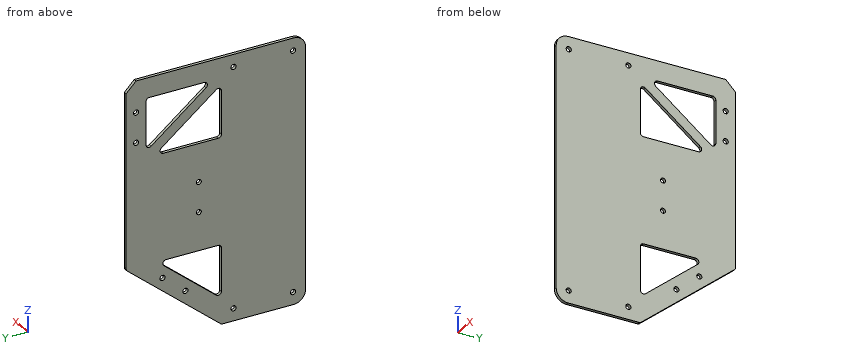
Autodesk Inventor part; units mm, degrees
ref_plane "YZ Plane" through (0, 0, 0) normal (1, 0, 0) x (0, 1, 0)
ref_plane "XZ Plane" through (0, 0, 0) normal (0, 1, 0) x (-1, 0, 0)
ref_plane "XY Plane" through (0, 0, 0) normal (0, 0, 1) x (1, 0, 0)
sketch "Sketch1" plane through (0, 0, 0) normal (1, 0, 0) x (0, 1, 0)
  line L0 (0, 0) -> (40, 0) construction
  line L1 (40, 0) -> (40, 66.5) construction
  line L2 (40, 66.5) -> (0, 66.5) construction
  line L3 (0, 66.5) -> (0, 0) construction
  line L4 (0, 66.5) -> (40, 66.5) construction
  line L5 (40, 66.5) -> (40, 86.5) construction
  line L6 (40, 86.5) -> (0, 86.5)
  line L7 (0, 86.5) -> (0, 66.5) construction
  line L8 (0, 0) -> (40, 0) construction
  line L9 (40, 0) -> (40, -20) construction
  line L10 (40, -20) -> (0, -20) construction
  line L11 (0, -20) -> (0, 0) construction
  line L12 (48.2, 61.45) -> (-8.2, 61.45) construction
  line L13 (-8.2, 61.45) -> (-8.2, 5.05) construction
  line L14 (-8.2, 5.05) -> (48.2, 5.05) construction
  line L15 (48.2, 5.05) -> (48.2, 61.45) construction
  line L16 (48.2, 33.25) -> (-8.2, 33.25) construction
  line L17 (40, 33.25) -> (0, 33.25) construction
  line L18 (43.57, 56.82) -> (-3.57, 56.82) construction
  line L19 (-3.57, 56.82) -> (-3.57, 9.68) construction
  line L20 (-3.57, 9.68) -> (43.57, 9.68) construction
  line L21 (43.57, 9.68) -> (43.57, 56.82) construction
  line L22 (43.57, 56.82) -> (48.2, 56.82) construction
  line L23 (43.57, 56.82) -> (43.57, 61.45) construction
  line L24 (-3.57, 9.68) -> (-8.2, 9.68) construction
  line L25 (-3.57, 9.68) -> (-3.57, 5.05) construction
  line L26 (40, -10) -> (0, -10) construction
  line L27 (40, 76.5) -> (0, 76.5) construction
  circle A0 centre (30, 76.5) radius 2.1
  circle A1 centre (10, 76.5) radius 2.1
  circle A2 centre (30, -10) radius 2.1
  circle A3 centre (10, -10) radius 2.1
  circle A4 centre (43.57, 56.82) radius 2.6
  circle A5 centre (43.57, 9.68) radius 2.6
  circle A6 centre (-3.57, 9.68) radius 2.6
  circle A7 centre (-3.57, 56.82) radius 2.6
  circle A8 centre (20, 33.25) radius 19.15
  circle A9 centre (-25, 18.25) radius 11.08 construction
  circle A10 centre (-25, 18.25) radius 13 construction
  circle A11 centre (-25, 18.25) radius 2.5
  line L28 (-60, 153.25) -> (-60, -86.75) construction
  circle A12 centre (-60, -86.75) radius 2.6
  circle A13 centre (-60, 153.25) radius 2.6
  line L29 (-120.2, 153.25) -> (-120.2, -86.75) construction
  circle A14 centre (-120.2, -86.75) radius 2.6
  circle A15 centre (-120.2, 153.25) radius 2.6
  circle A16 centre (-60, -86.75) radius 12 construction
  circle A17 centre (-120.2, -86.75) radius 12 construction
  circle A18 centre (-120.2, 153.25) radius 12 construction
  circle A19 centre (-60, 153.25) radius 12 construction
  line L30 (-110, 482.7599) -> (-70, 482.7599) construction
  line L31 (-70, -517.2401) -> (-110, -517.2401) construction
  circle A20 centre (-25, 48.25) radius 2.5
  circle A21 centre (-25, 48.25) radius 11.08 construction
  circle A22 centre (-25, 48.25) radius 13 construction
  circle A23 centre (20, 33.25) radius 11.08 construction
  circle A24 centre (20, 33.25) radius 13 construction
  line L32 (-23.1873, 29.1807) -> (18.1873, 22.3193) construction
  line L33 (18.1873, 44.1807) -> (-23.1873, 37.3193) construction
  line L34 (-120.8333, -99.25) -> (-47.8333, -99.25)
  line L35 (-47.8333, 165.75) -> (-120.8333, 165.75)
  line L36 (-132.8333, 153.75) -> (-132.8333, -87.25)
  line L37 (-60, 153.25) -> (-120.2, 153.25) construction
  line L38 (-120.2, -86.75) -> (-60, -86.75) construction
  line L39 (-60, 153.25) -> (-60, 165.75) construction
  line L40 (-120.2, -86.75) -> (-120.2, -99.25) construction
  line L41 (48.3276, -20) -> (48.3276, 86.5)
  line L42 (17.6122, 86.5) -> (40, 86.5) construction
  arc A25 (-120.8333, 165.75) -> (-132.8333, 153.75) centre (-120.8333, 153.75) ccw
  arc A26 (-132.8333, -87.25) -> (-120.8333, -99.25) centre (-120.8333, -87.25) ccw
  line L43 (48.3276, -20) -> (-47.8333, -99.25)
  line L44 (-47.8333, 165.75) -> (-47.8333, -99.25) construction
  line L45 (-120.2, -86.75) -> (-132.8333, -86.75) construction
  line L46 (-60, 153.25) -> (-47.8333, 153.25) construction
  line L47 (-36.08, 48.25) -> (-36.08, 286.613) construction
  line L48 (-47.8333, 145.75) -> (-47.8333, 86.5)
  line L49 (-47.8333, 86.5) -> (16.8804, 86.5)
  line L50 (-47.8333, -73.3332) -> (16.8804, -20)
  line L51 (-47.8333, -20) -> (16.8804, -20)
  line L52 (-47.8333, -73.3332) -> (-47.8333, -20)
  line L53 (48.3276, 86.5) -> (48.3276, 165.75)
  line L54 (48.3276, 165.75) -> (-47.8333, 165.75)
  line L55 (-47.8333, 145.75) -> (28.3276, 145.75)
  line L56 (28.3276, 145.75) -> (28.3276, 86.5)
  line L57 (-47.8333, 145.75) -> (28.3276, 86.5) construction
  line L58 (-39.6904, 145.75) -> (28.3276, 92.8349)
  line L59 (-47.8333, 139.4151) -> (20.1847, 86.5)
  point P0 (-132.8333, -99.25)
  point P1 (-132.8333, 165.75)
  point P2 (-47.8333, 139.8332)
  point P3 (0, 86.5)
  point P4 (0, 86.5)
  dimension "d190" = 22.16
  dimension "d165" = 40
  dimension "d166" = 66.5
  dimension "d167" = 40
  dimension "d168" = 20
  dimension "d169" = 40
  dimension "d170" = 20
  dimension "d171" = 56.4
  dimension "d172" = 56.4
  dimension "d173" = 0
  dimension "d174" = 8.2
  dimension "d175" = 47.14
  dimension "d176" = 47.14
  dimension "d177" = 4.2
  dimension "d178" = 20
  dimension "d179" = 10
  dimension "d180" = 10
  dimension "d181" = 20
  dimension "d182" = 4.2
  dimension "d183" = 4.2
  dimension "d184" = 4.2
  dimension "d185" = 5.2
  dimension "d186" = 5.2
  dimension "d187" = 5.2
  dimension "d188" = 5.2
  dimension "d189" = 38.3
  dimension "d191" = 26
  dimension "d192" = 5
  dimension "d193" = 240
  dimension "d194" = 60
  dimension "d195" = 5.2
  dimension "d196" = 5.2
  dimension "d197" = 5.2
  dimension "d198" = 5.2
  dimension "d199" = 60.2
  dimension "d200" = 24
  dimension "d201" = 24
  dimension "d202" = 24
  dimension "d203" = 24
  dimension "d204" = 40
  dimension "d205" = 1000
  dimension "d206" = 45
  dimension "d207" = 5
  dimension "d208" = 22.16
  dimension "d209" = 26
  dimension "d210" = 45
  dimension "d211" = 22.16
  dimension "d212" = 26
  dimension "d213" = 15
  dimension "d214" = 15
  dimension "d215" = 265
  dimension "d216" = 85
  dimension "d217" = 106.5
  dimension "d218" = 12
  dimension "d219" = 72.8333
  dimension "d220" = 28.3276
  dimension "d221" = 53.25
  dimension "d222" = 85
  dimension "d223" = 132.5
  dimension "d224" = 60.2
  dimension "d225" = 20
  dimension "d226" = 20
  dimension "d227" = 5
  dimension "d228" = 5
extrude "Extrusion1" add sketch "Sketch1" along normal blind 3.175 contours L6 L59 L48 L55 L58 L56 | A0 | A1 | A2 | A3 | A4 | A5 | A6 | A7 | A8 | A26 L36 A25 L35 L54 L53 L41 L43 L34
sketch "Sketch6" plane through (3.175, 0, 0) normal (1, 0, 0) x (0, 0, -1)
  line L0 (20, 16.8804) -> (73.3332, -47.8333)
  line L1 (20, 16.8804) -> (73.3332, -47.8333)
  line L2 (39.0796, -6.2705) -> (54.5136, 6.4492) construction
  line L3 (99.25, -47.8333) -> (20, 48.3276)
  circle A0 centre (37.2568, 11.6648) radius 2.6
  circle A1 centre (56.3364, -11.4861) radius 2.6
  line L4 (37.2568, 11.6648) -> (46.7966, 0.0893) construction
  line L5 (56.3364, -11.4861) -> (46.7966, 0.0893) construction
  line L6 (-145.75, 28.3276) -> (-92.8349, 28.3276)
  line L7 (-119.2924, 28.3276) -> (-119.2924, 48.3276) construction
  line L8 (20, 48.3276) -> (-165.75, 48.3276) construction
  circle A2 centre (-104.2924, 38.3276) radius 2.6
  circle A3 centre (-134.2924, 38.3276) radius 2.6
  line L9 (-104.2924, 38.3276) -> (-119.2924, 38.3276) construction
  line L10 (-134.2924, 38.3276) -> (-119.2924, 38.3276) construction
  point P0 (0, 0)
  dimension "d229" = 5.2
  dimension "d230" = 5.2
  dimension "d231" = 15
  dimension "d232" = 15
  dimension "d233" = 30
  dimension "d234" = 5.2
  dimension "d235" = 5.2
  dimension "d236" = 15
  dimension "d237" = 15
extrude "Extrusion6" cut sketch "Sketch6" against normal through all
fillet "Fillet2" radius 3.175 11 edges at (1.5875, 28.3276, 92.8349) (1.5875, 20.1847, 86.5) (1.5875, 28.3276, 145.75) (1.5875, -39.6904, 145.75) (1.5875, -47.8333, 139.4151) (1.5875, -47.8333, 86.5) (1.5875, 48.3276, -20) (1.5875, 16.8804, -20) (1.5875, -47.8333, -20) (1.5875, -47.8333, -73.3332) (1.5875, -47.8333, -99.25)
chamfer "Chamfer1" distance 10 angle 45 1 edges at (1.5875, 48.3276, 165.75)
properties part number "X Axis Belt V Wheel LEFT Outside Frame Machined No Logo"
Verification items for the finished model (mm, model axes). Round coordinates to 2 decimals unless told otherwise and drop trailing zeros. Order: outer loops, then holes, each group sorted by start corner. A loop starts at its lowest first (then second) coordinate and runs counter-clockwise, first axis right, second up.
1. Section check C-C on x = 2.3. State how many separate pieces and enclosed holes the cut face has, then the cut area to 3 significant figures.
Final values:
separate pieces: 1
enclosed holes: 13
area: 38,600 mm2
2. Go/stop test with flat-tipped pins: P1, Ø1.5, axis at x = 1, y = -16, coming from the -Z side; P2, Ø1.6, axis at x = 1, z = -44, coming from the +Y side. Record where each tip stops, or that it passes through.
Final values:
P1: stops at z = -73.63
P2: stops at y = 20.18
3. Section check A-A on y = -60. Record the cut outline in (x, z) (3 decimals).
Final values:
outline: (0, -99.25) - (3.175, -99.25) - (3.175, -89.35) - (0, -89.35) - close; (0, -84.15) - (3.175, -84.15) - (3.175, 150.65) - (0, 150.65) - close; (0, 155.85) - (3.175, 155.85) - (3.175, 165.75) - (0, 165.75) - close
4. Thickness scan on L1, parallel to Z at x = 1.55, y = -60; L2, parallel to Z at x = 2.4, y = -34; L3, parallel to Z at x = 1.9, y = -4.5. Record the ranges inside material, lowest first.
Final values:
L1: z = -99.25 to -89.35, -84.15 to 150.65, 155.85 to 165.75
L2: z = -87.85 to -61.93, -20 to 86.5, 128.65 to 165.75
L3: z = -63.54 to -37.62, -20 to 86.5, 105.7 to 118.37, 145.75 to 165.75
5. Section check B-B on y = -4. Record the cut outline in (x, z) (3 decimals).
Final values:
outline: (0, -63.125) - (3.175, -63.125) - (3.175, -37.208) - (0, -37.208) - close; (0, -20) - (3.175, -20) - (3.175, 86.5) - (0, 86.5) - close; (0, 105.315) - (3.175, 105.315) - (3.175, 117.984) - (0, 117.984) - close; (0, 145.75) - (3.175, 145.75) - (3.175, 165.75) - (0, 165.75) - close
